Part model, mm, in its own coordinate system. Face numbers are marked on the shaded views. A direction names the side the tool comes from. Round coordinates to 2 decimals unless told otherwise and drop trailing zeros. Write each loop counter-clockwise with the first axis right and the second up, starting at its lowest first coordinate (ties: lowest second). Pieces come first, ordered by that corner, then holes.
1) Saw through at A-A on x = 0. Write the cut outline in (y, z) (3 decimals), and give its area (3 significant figures).
2) Drill centre lines: L1, parallel to Y at x = 0, z = 26.5; L2, parallel to Z at x = 7.75, y = 2.5 (3 decimals); L3, parallel to Y at x = 0, z = 11. Where is each one in solid material? Low to high.
3) Saw through at C-C on z = 28. Write the cut outline in (x, y), and give its area (3 significant figures).
4) Which spindle directions (+Z, -Z, +X, -X, +Y, -Y) get a long thin tool onto all of the face, cutting with end or side? Do the marked faces 4 and 5. Say none if no direction does.
5) Flat gauge pins, fed straight in: pin 1 (4 mm diameter, centred on x = -4.5, z = 25, fed in from -Y); pin 2 (2 mm diameter, centred on y = -3.5, z = 12, fed in from -X); pin 3 (5 mm diameter, centred on x = 7.5, z = 41.5, fed in from +Y). Where does each tip first touch, or does it go through?
6) Saw through at D-D on z = 7. Write the cut outline in (x, y), and give its area (3 significant figures).
7) Pull direction Y, two halves, no side cores. Call the marked faces 1, 2 and 3: +Y half, -Y half, draft (parallel to the pull), parting line (faces both ways), or undercut.
```python
from build123d import *

# Parameters (mm, degrees)
F0_R     = 12.7
F1_DEPTH = 50.8
F2_W     = 5.08
F2_H     = 9.525
F4_SIZE  = 2.54
F6_D     = 5.1054


with BuildPart() as f1:
    # F0 (on Top) → F1 (new body)
    with BuildSketch(Plane.XY):
        Circle(F0_R)
    extrude(amount=F1_DEPTH)

    # F2 (on Right) → F3 (revolve, cut)
    with BuildSketch(Plane.YZ):
        with Locations((-10.16, 30.1625)):
            Rectangle(F2_W, F2_H)
    revolve(axis=Axis((0, 0, 51.1521063745), (0, 0, -1)), mode=Mode.SUBTRACT)

    # F4
    f4_edges = [f1.edges().sort_by_distance(p)[0] for p in [
        (-12.7, 0, 25.4),
        (-12.7, 0, 34.925),
    ]]
    chamfer(f4_edges, length=F4_SIZE)

    # F6 (through all)
    with Locations(Plane(origin=(0, 0, 0), x_dir=(1, 0, 0), z_dir=(0, 0, -1))):
        with Locations((0, 0)):
            Hole(F6_D / 2)


solid = f1.part
```
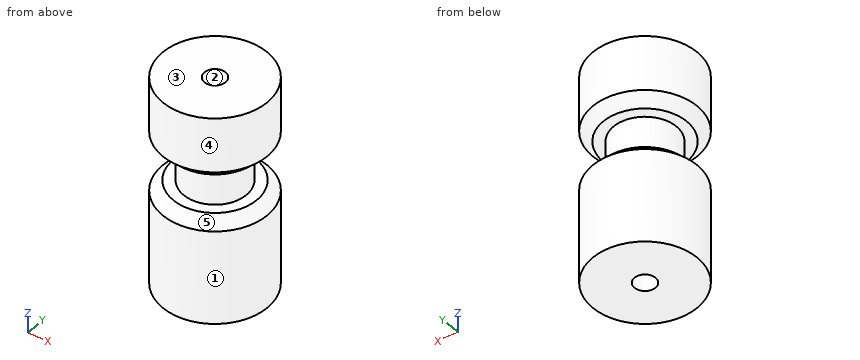
Completed:
1. outline: (-12.7, 0) - (-2.553, 0) - (-2.553, 50.8) - (-12.7, 50.8) - (-12.7, 37.465) - (-10.16, 34.925) - (-7.62, 34.925) - (-7.62, 25.4) - (-10.16, 25.4) - (-12.7, 22.86) - close; (2.553, 0) - (12.7, 0) - (12.7, 22.86) - (10.16, 25.4) - (7.62, 25.4) - (7.62, 34.925) - (10.16, 34.925) - (12.7, 37.465) - (12.7, 50.8) - (2.553, 50.8) - close
1. area: 921 mm2
2. L1: y = -7.62 to -2.55, 2.55 to 7.62
2. L2: z = 0 to 25.4, 34.925 to 50.8
2. L3: y = -12.7 to -2.55, 2.55 to 12.7
3. outline: circle Ø15.24 at (0, 0); hole circle Ø5.11 at (0, 0)
3. area: 162 mm2
4. face 4: +Z, -Z
4. face 5: none
5. pin 1: stops at y = -11.84
5. pin 2: stops at x = -12.45
5. pin 3: stops at y = 11.67
6. outline: circle Ø25.4 at (0, 0); hole circle Ø5.11 at (0, 0)
6. area: 486 mm2
7. face 1: parting line
7. face 2: undercut
7. face 3: draft
